Part model, mm, in its own coordinate system. Face numbers are marked on the shaded views. A direction names the side the tool comes from. Round coordinates to 2 decimals unless told otherwise and drop trailing zeros. Loops run counter-clockwise (first coordinate to the right, second up) from the corner with the lowest first, then second, coordinate; pieces in that order, holes last. Notation, with made-up numbers: M 79,-13 L 116,-13 A31 ccw 116,15 Z; hole C -24,27 d1. An arc over 180 degrees is marked long. Put each result on its own line as item: value. Start each with the question number.
1) Drop a flat-ended pin along its axis: pin 1 Ø3.5 at (x, y) = (31.75, 0) entering from +Z. Give the stop position or say it passes through.
2) Probe line 1 along X through (y, z) = (-23.9, 0); line 2 along Z through (x, y) = (9, -16.5); line 3 along Y through (x, z) = (41.5, 8.25). List the from-to ranges inside material, lowest first.
3) Slice it at B-B on z = 7.75. Give the cut face in (x, y), then the cut area to 3 significant figures.
4) Slice it at A-A on x = 6.35. Give the cut face in (y, z), then the cut area to 3 significant figures.
5) Slice it at D-D on x = 34.5. Give the cut face in (y, z), then the cut area to 3 significant figures.
6) Slice it at C-C on y = 0. State how many separate pieces and enclosed holes the cut face has, then the cut area to 3 significant figures.
7) Which spindle directions (+Z, -Z, +X, -X, +Y, -Y) get a long thin tool onto all of the face, cutting with end or side? Do the marked faces 1 and 2. Say none if no direction does.
8) Pull direction Z, two halves, no side cores. Call the marked faces 3, 4 and 5: +Z half, -Z half, draft (parallel to the pull), parting line (faces both ways), or undercut.
```python
from build123d import *

# Parameters (mm, degrees)
SKETCH1_W           = 25.4
SKETCH1_H           = 50.8
SKETCH1_W_2         = 20.32
SKETCH1_H_2         = 45.72
BOSS_EXTRUDE1_DEPTH = 44.45
SKETCH4_R           = 2.032
CUT_EXTRUDE3_DEPTH  = 69.685751798
SKETCH6_R           = 2.032
CUT_EXTRUDE5_DEPTH  = 58.15


with BuildPart() as part:
    # Sketch1 → Boss-Extrude1 (new body)
    with BuildSketch(Plane(origin=(0, 0, 0), x_dir=(0, 0, -1), z_dir=(1, 0, 0))):
        Rectangle(SKETCH1_W, SKETCH1_H)
        Rectangle(SKETCH1_W_2, SKETCH1_H_2, mode=Mode.SUBTRACT)
    extrude(amount=BOSS_EXTRUDE1_DEPTH)

    # Sketch4 → Cut-Extrude3 (cut, through all)
    with BuildSketch(Plane.XZ.offset(25.4)):
        with Locations(Location((6.35, 0, 0), (0, 0, 270))):
            Circle(SKETCH4_R)
        with Locations(Location((19.05, 0, 0), (0, 0, 270))):
            Circle(SKETCH4_R)
        with Locations(Location((31.75, 0, 0), (0, 0, 270))):
            Circle(SKETCH4_R)
        with Locations((44.45, 0)):
            Circle(SKETCH4_R)
        with Locations((57.15, 0)):
            Circle(SKETCH4_R)
        with Locations((69.85, 0)):
            Circle(SKETCH4_R)
    extrude(amount=-CUT_EXTRUDE3_DEPTH, mode=Mode.SUBTRACT)

    # Sketch6 → Cut-Extrude5 (cut, through all)
    with BuildSketch(Plane(origin=(0, 0, -12.7), x_dir=(-1, 0, 0), z_dir=(0, 0, -1))):
        with Locations((-44.45, 0)):
            Circle(SKETCH6_R)
        with Locations((-31.75, 0)):
            Circle(SKETCH6_R)
        with Locations((-19.05, 0)):
            Circle(SKETCH6_R)
        with Locations((-6.35, 0)):
            Circle(SKETCH6_R)
        with Locations((6.35, 0)):
            Circle(SKETCH6_R)
        with Locations((19.05, 0)):
            Circle(SKETCH6_R)
        with Locations((31.75, 0)):
            Circle(SKETCH6_R)
    extrude(amount=-CUT_EXTRUDE5_DEPTH, mode=Mode.SUBTRACT)


solid = part.part
```
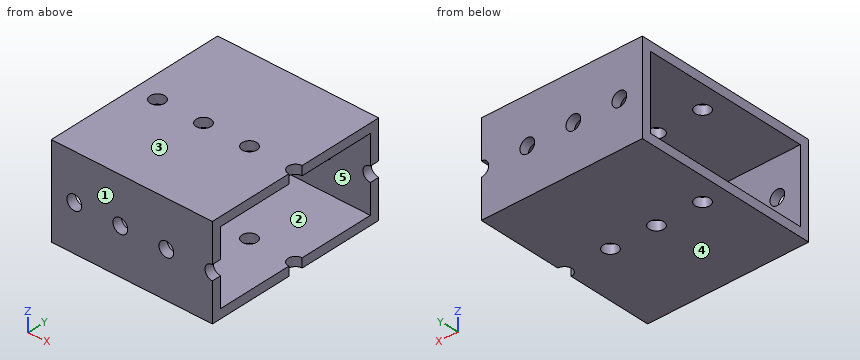
Recorded:
1. pin 1: passes through
2. line 1: x = 0 to 4.32, 8.38 to 17.02, 21.08 to 29.72, 33.78 to 42.42
2. line 2: z = -12.7 to -10.16, 10.16 to 12.7
2. line 3: y = -25.4 to -22.86, 22.86 to 25.4
3. outline: M 0,-25.4 L 44.45,-25.4 L 44.45,-22.86 L 0,-22.86 Z; M 0,22.86 L 44.45,22.86 L 44.45,25.4 L 0,25.4 Z
3. area: 226 mm2
4. outline: M -25.4,-12.7 L -2.03,-12.7 L -2.03,-10.16 L -22.86,-10.16 L -22.86,-2.03 L -25.4,-2.03 Z; M -25.4,2.03 L -22.86,2.03 L -22.86,10.16 L -2.03,10.16 L -2.03,12.7 L -25.4,12.7 Z; M 2.03,-12.7 L 25.4,-12.7 L 25.4,-2.03 L 22.86,-2.03 L 22.86,-10.16 L 2.03,-10.16 Z; M 2.03,10.16 L 22.86,10.16 L 22.86,2.03 L 25.4,2.03 L 25.4,12.7 L 2.03,12.7 Z
4. area: 320 mm2
5. outline: M -25.4,-12.7 L 25.4,-12.7 L 25.4,12.7 L -25.4,12.7 Z; hole M -22.86,-10.16 L 22.86,-10.16 L 22.86,10.16 L -22.86,10.16 Z
5. area: 361 mm2
6. separate pieces: 8
6. enclosed holes: 0
6. area: 154 mm2
7. face 1: +Z, -Z, +X, -X, -Y
7. face 2: +X, -X
8. face 3: +Z half
8. face 4: -Z half
8. face 5: undercut
